Here's how the part is built. I have some questions about the finished solid (model axes, mm). A direction names the side the tool comes from. Give positions to 0.01 mm unless a question says otherwise; leave off trailing zeros. Loops run counter-clockwise (first coordinate to the right, second up) from the corner with the lowest first, then second, coordinate; pieces in that order, holes last. Notation, with made-up numbers: (-17, -24.5) - (13, -24.5) arc R21 cw to (13, -9.5) - close; hole circle Ø9 at (35, -5). An arc over 180 degrees is marked (long way). Use one line per item in the form item = value.
from build123d import *

# Parameters (mm, degrees)
SKETCH1_R           = 8.149999999999999
BOSS_EXTRUDE1_DEPTH = 6
BOSS_EXTRUDE2_DEPTH = 1.1
BOSS_EXTRUDE3_DEPTH = 0.8
SKETCH4_R           = 5.35
BOSS_EXTRUDE4_DEPTH = 1
SKETCH5_R           = 3.35
BOSS_EXTRUDE5_DEPTH = 6.4
FILLET1_R           = 1
SKETCH6_R           = 2.9
BOSS_EXTRUDE6_DEPTH = 12.8
CUT_EXTRUDE1_DEPTH  = 11.3
FILLET2_R           = 1


with BuildPart() as part:
    # Sketch1 → Boss-Extrude1 (new body)
    with BuildSketch(Plane(origin=(0, 0, 0), x_dir=(1, 0, 0), z_dir=(0, 1, 0))):
        with Locations(Location((0, 0, 0), (0, 0, 270))):
            Circle(SKETCH1_R)
    extrude(amount=BOSS_EXTRUDE1_DEPTH)

    # Sketch2 → Boss-Extrude2 (add)
    with BuildSketch(Plane(origin=(0, 6, 0), x_dir=(1, 0, 0), z_dir=(0, 1, 0))):
        with BuildLine():
            Line((0, -8.15), (11.85, -8.15))
            Line((11.85, -8.15), (11.849999999999996, 8.150000000000004))
            Line((11.849999999999996, 8.150000000000004), (0, 8.15))
            ThreePointArc((0, 8.15), (-8.15, 1e-15), (0, -8.15))
        make_face()
    extrude(amount=BOSS_EXTRUDE2_DEPTH)

    # Sketch3 → Boss-Extrude3 (add)
    with BuildSketch(Plane(origin=(0, 7.1000000000000005, 0), x_dir=(1, 0, 0), z_dir=(0, 1, 0))):
        with BuildLine():
            Line((-5.45, 6.059702963017249), (-5.45, -6.059702963017249))
            ThreePointArc((-5.45, -6.059702963017249), (-1.31e-15, -8.150000000000002), (5.45, -6.059702963017249))
            Line((5.45, -6.059702963017249), (5.45, 6.059702963017249))
            ThreePointArc((5.45, 6.059702963017249), (5e-16, 8.150000000000002), (-5.45, 6.059702963017249))
        make_face()
    extrude(amount=BOSS_EXTRUDE3_DEPTH)

    # Sketch4 → Boss-Extrude4 (add)
    with BuildSketch(Plane(origin=(0, 7.9, 0), x_dir=(1, 0, 0), z_dir=(0, 1, 0))):
        with Locations(Location((0, 0, 0), (0, 0, 270))):
            Circle(SKETCH4_R)
    extrude(amount=BOSS_EXTRUDE4_DEPTH)

    # Sketch5 → Boss-Extrude5 (add)
    with BuildSketch(Plane(origin=(0, 8.900000000000002, 0), x_dir=(1, 0, 0), z_dir=(0, 1, 0))):
        with Locations(Location((0, 0, 0), (0, 0, 270))):
            Circle(SKETCH5_R)
    extrude(amount=BOSS_EXTRUDE5_DEPTH)

    # Fillet1
    fillet1_edges = [part.edges().sort_by_distance(p)[0] for p in [
        (2.5e-15, 0, -8.149999999999999),
        (1.03e-15, 15.300000000000002, -3.35),
    ]]
    fillet(fillet1_edges, radius=FILLET1_R)

    # Sketch6 → Boss-Extrude6 (add)
    with BuildSketch(Plane(origin=(0, 15.3, 0), x_dir=(1, 0, 0), z_dir=(0, 1, 0))):
        with Locations(Location((0, 0, 0), (0, 0, 270))):
            Circle(SKETCH6_R)
    extrude(amount=BOSS_EXTRUDE6_DEPTH)

    # Sketch7 → Cut-Extrude1 (cut)
    with BuildSketch(Plane(origin=(0, 28.1, 0), x_dir=(1, 0, 0), z_dir=(0, 1, 0))):
        Polygon((0.5499999999999995, 5.000000000000001), (-0.5500000000000006, 5.000000000000001), (-0.5499999999999994, -4.999999999999999), (0.5500000000000007, -4.999999999999999), align=None)
    extrude(amount=-CUT_EXTRUDE1_DEPTH, mode=Mode.SUBTRACT)

    # Fillet2
    fillet2_edges = [part.edges().sort_by_distance(p)[0] for p in [
        (2.9, 28.1, 7.347e-14),
        (-2.9, 28.1, 7.105e-14),
    ]]
    fillet(fillet2_edges, radius=FILLET2_R)


solid = part.part
(1) If we section it at C-C (y = 7.5): List the corners of the cut face in (x, z) for me, plus the area to 3 significant figures.
Geometry says:
outline = (-5.45, -6.06) arc R8.15 ccw to (5.45, -6.06) - (5.45, 6.06) arc R8.15 ccw to (-5.45, 6.06) - close
area = 163 mm²
(2) If we section it at A-A (y = 17.5): List the corners of the cut face in (x, z) for me.
Geometry says:
outline = (-0.55, -2.85) - (-0.55, 2.85) arc R2.9 ccw to start; (0.55, -2.85) arc R2.9 ccw to (0.55, 2.85) - close
(3) For faces 1 (the flat face through (-7, 7.1, 0)), 2 (the cylindrical face through (0.871, 21.117, 2.766)), 3 (the flat face through (0.55, 23, 0)), which set-ups out of +Z, -Z, +X, -X, +Y, -Y let a thin tool reach every point of the face, with its end or its side?
Geometry says:
face_1 = +Z, -Z, -X, +Y
face_2 = +Y
face_3 = +Z, -Z, +Y
(4) For P1, Ø6, axis at x = -5.5, y = 8.5, coming from the +Z side; P2, Ø4, axis at y = 19.5, z = -0.5, coming from the -X side; P3, Ø1.5, axis at y = 15, z = 1.5, coming from the +X side, each with a flat end and sliding along its axis, tell me the tip position at first contact or that it passes through.
Geometry says:
P1 = 7.74
P2 = -2.9
P3 = 3.19
(5) If I drill on probe 1 along X at (y, z) = (21.25, 0); probe 2 along Y at (x, z) = (6, 7); probe 3 along Y at (x, z) = (5.75, -1.75), over which ranges is the centre line in solid material (lowest first)?
Geometry says:
probe_1 = -2.9 to -0.55, 0.55 to 2.9
probe_2 = 6 to 7.1
probe_3 = 0 to 7.1
(6) Thinking about a two-plate mould opening in X: for faces 4 (the cylindrical face through (-5.223, 8.393, -1.16)), 5 (the flat face through (0, 16.8, 0)), 6 (the flat face through (11.85, 6.5, 0.1)), 7 (the flat face through (2.3, 7.9, 5.3)), which applies, pulls with the +X half, pulls with the -X half, needs draft (parallel to the pull), parting line crosses it, or undercut?
Geometry says:
face_4 = parting line crosses it
face_5 = undercut
face_6 = pulls with the +X half
face_7 = needs draft
